from build123d import *

# Parameters (mm, degrees)
F1_DEPTH = 19.05
F2_W     = 406.4
F2_H     = 3.175
F3_DEPTH = 17.4625
F4_W     = 406.4
F4_H     = 31.75
F5_DEPTH = 12.7


with BuildPart() as f1:
    # F0 (on Front) → F1 (new body)
    with BuildSketch(Plane.XZ):
        Polygon((218.022645, -71.199347), (218.022645, 487.600653), (243.422645, 487.600653), (243.422645, 538.400653), (-213.777355, 538.400653), (-213.777355, 487.600653), (-188.377355, 487.600653), (-188.377355, -71.199347), align=None)
    extrude(amount=F1_DEPTH)

    # F2 (on face) → F3 (cut)
    with BuildSketch(Plane.XZ.offset(19.05)):
        with Locations((14.822645, 257.413153)):
            Rectangle(F2_W, F2_H)
        with Locations((14.822645, 229.790653)):
            Rectangle(F2_W, F2_H)
        with Locations((14.822645, 254.238153)):
            Rectangle(F2_W, F2_H)
        with Locations((14.822645, 202.168153)):
            Rectangle(F2_W, F2_H)
        with Locations((14.822645, 174.545653)):
            Rectangle(F2_W, F2_H)
        with Locations((14.822645, 146.923153)):
            Rectangle(F2_W, F2_H)
        with Locations((14.822645, 119.300653)):
            Rectangle(F2_W, F2_H)
        with Locations((14.822645, 91.678153)):
            Rectangle(F2_W, F2_H)
        with Locations((14.822645, 64.055653)):
            Rectangle(F2_W, F2_H)
        with Locations((14.822645, 36.433153)):
            Rectangle(F2_W, F2_H)
        with Locations((14.822645, 8.810653)):
            Rectangle(F2_W, F2_H)
        with Locations((14.822645, -18.811847)):
            Rectangle(F2_W, F2_H)
    extrude(amount=-F3_DEPTH, mode=Mode.SUBTRACT)

    # F4 (on face) → F5 (cut)
    with BuildSketch(Plane(origin=(0, 0, 0), x_dir=(-1, 0, 0), z_dir=(0, 1, 0))):
        with Locations((-14.822645, -55.324347)):
            Rectangle(F4_W, F4_H)
    extrude(amount=-F5_DEPTH, mode=Mode.SUBTRACT)


solid = f1.part
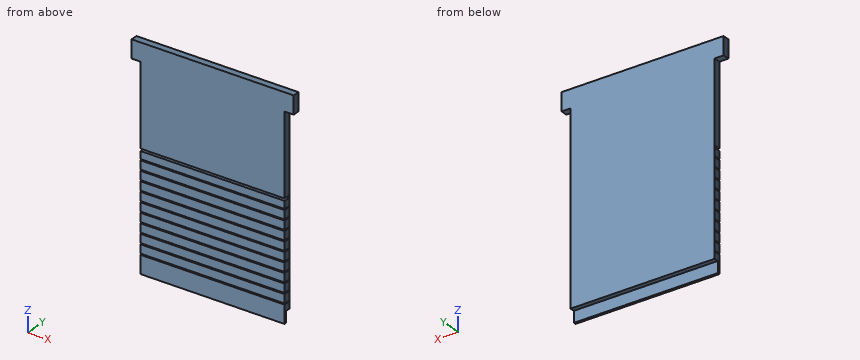
Geometry: final body of the model. Coordinates: model frame, mm. Give positions to 0.01 mm unless a question says otherwise; leave off trailing zeros. Order: outer loops, then holes, each group sorted by start corner. A loop starts at its lowest first (then second) coordinate and runs counter-clockwise, first axis right, second up. Notation, with made-up numbers: (60, 56) -> (103, 56) arc R19 ccw to (103, 86) -> close; hole circle Ø8 at (45.25, -31.5). An arc over 180 degrees is marked (long way). Write each question's results on one line, items separated by ' | '.
1) Cut plane A-A (y = -16). Give the number of separate pieces and of enclosed holes in the cut face, and give its area (3 significant figures).
Geometry says:
separate pieces: 12 | enclosed holes: 0 | area: 235,000 mm²
2) First-contact query: pin 1 Ø1 at (x, z) = (90, 36) entering from -Y; pin 2 Ø3 at (y, z) = (-6, 290.5) entering from -X; pin 3 Ø5.5 at (x, y) = (231, -8.5) entering from -Z. Flat tips, straight axial feed; report the tip coordinate or a pass-through.
Geometry says:
pin 1: stops at y = -1.59 | pin 2: stops at x = -188.38 | pin 3: stops at z = 487.6
3) Line query: line 1 along X through (y, z) = (-5.5, 388); line 2 along Z through (x, y) = (-189.5, -5.25). Output: solid intervals per line, ascending.
Geometry says:
line 1: x = -188.38 to 218.02 | line 2: z = 487.6 to 538.4
4) Cut plane B-B (z = 282.5). Output: boundary loops of the cut face in (x, y).
Geometry says:
outline: (-188.38, -19.05) -> (218.02, -19.05) -> (218.02, 0) -> (-188.38, 0) -> close
